The model under review builds one solid part; all positions refer to its coordinate system, in mm. Face numbers are marked on the shaded views. A direction names the side the tool comes from. Round coordinates to 2 decimals unless told otherwise and drop trailing zeros. Order: outer loops, then holes, each group sorted by start corner. A loop starts at its lowest first (then second) coordinate and runs counter-clockwise, first axis right, second up. Notation, with made-up numbers: M -40,87 L 14,87 A32 cw 14,117 Z; hole C -19.5,18 d4. An arc over 180 degrees is marked long. Answer as a JSON object with one key per item and string values. Group by question number.
1. Clearance check with flat-ended pins moving along their axes: P1, Ø1, axis at y = 12, z = 11.5, coming from the -X side; P2, Ø5, axis at x = -23.5, z = 8, coming from the +Y side; P3, Ø1.5, axis at y = -3, z = 7, coming from the +X side. State where each tip first meets the part, or that it passes through.
2. Add section B-B on y = -21. State the section outline as (x, z) points.
3. Add section C-C on x = 22.5. State the section outline as (y, z) points, and give its area (3 significant figures).
4. Add section A-A on z = 4. State the section outline as (x, y) points, and give its area (3 significant figures).
5. Mouldability with a two-part tool opening along X and no side actions: class the marked faces 3, 4 and 5 as released by +X, released by -X, zero draft, split by the parting line, or undercut.
6. Machinability: for the marked faces 1 and 2, which of the approach directions +Z, -Z, +X, -X, +Y, -Y give a long, thin tool a straight path to every point of the face, cutting with its end or side? Answer none if there is none.
7. To check wall thickness, follow probe 1 along X at (y, z) = (-23.7, 16); probe 2 along Z at (x, y) = (22.5, -22); probe 3 along X at (y, z) = (5.5, 8.5). State the ranges of each line that lie inside material, in increasing order. Write a range as [from, to].
8. Add section D-D on x = 0. State the section outline as (y, z) points, and give its area (3 significant figures).
```python
from build123d import *

# Parameters (mm, degrees)
SKETCH_1_W          = 35
SKETCH_1_H          = 50
EXTRUDE_1_DEPTH     = 20
SKETCH_2_W          = 20
SKETCH_2_H          = 5
EXTRUDE_2_DEPTH     = 10
SKETCH_3_W          = 20
SKETCH_3_H          = 5
EXTRUDE_3_DEPTH     = 10
SKETCH_4_R          = 12
CUT_EXTRUDE_1_DEPTH = 20
SKETCH_5_R          = 1.5
CUT_EXTRUDE_2_DEPTH = 5
SKETCH_6_R          = 1.5
CUT_EXTRUDE_3_DEPTH = 5
SKETCH_7_R          = 1.5
CUT_EXTRUDE_4_DEPTH = 5
SKETCH_8_R          = 1.5
CUT_EXTRUDE_5_DEPTH = 5


with BuildPart() as part:
    # Эскиз1 → Бобышка-Вытянуть1 (new body)
    with BuildSketch(Plane.XY):
        Rectangle(SKETCH_1_W, SKETCH_1_H)
    extrude(amount=EXTRUDE_1_DEPTH)

    # Эскиз2 → Бобышка-Вытянуть2 (add)
    with BuildSketch(Plane(origin=(17.5, 0, 0), x_dir=(0, 0, -1), z_dir=(1, 0, 0))):
        with Locations((-10, -22.5)):
            Rectangle(SKETCH_2_W, SKETCH_2_H)
    extrude(amount=EXTRUDE_2_DEPTH)

    # Эскиз3 → Бобышка-Вытянуть3 (add)
    with BuildSketch(Plane.ZY.offset(17.5)):
        with Locations((10, -22.5)):
            Rectangle(SKETCH_3_W, SKETCH_3_H)
    extrude(amount=EXTRUDE_3_DEPTH)

    # Эскиз4 → Вырез-Вытянуть1 (cut)
    with BuildSketch(Plane(origin=(0, 0, 0), x_dir=(-1, 0, 0), z_dir=(0, 0, -1))):
        with Locations((0, 5)):
            Circle(SKETCH_4_R)
    extrude(amount=-CUT_EXTRUDE_1_DEPTH, mode=Mode.SUBTRACT)

    # Эскиз5 → Вырез-Вытянуть2 (cut)
    with BuildSketch(Plane(origin=(0, -20, 0), x_dir=(1, 0, 0), z_dir=(0, 1, 0))):
        with Locations((-22.5, -4)):
            Circle(SKETCH_5_R)
    extrude(amount=-CUT_EXTRUDE_2_DEPTH, mode=Mode.SUBTRACT)

    # Эскиз6 → Вырез-Вытянуть3 (cut)
    with BuildSketch(Plane(origin=(0, -20, 0), x_dir=(1, 0, 0), z_dir=(0, 1, 0))):
        with Locations((-22.5, -16)):
            Circle(SKETCH_6_R)
    extrude(amount=-CUT_EXTRUDE_3_DEPTH, mode=Mode.SUBTRACT)

    # Эскиз7 → Вырез-Вытянуть4 (cut)
    with BuildSketch(Plane(origin=(0, -20, 0), x_dir=(1, 0, 0), z_dir=(0, 1, 0))):
        with Locations((22.5, -4)):
            Circle(SKETCH_7_R)
    extrude(amount=-CUT_EXTRUDE_4_DEPTH, mode=Mode.SUBTRACT)

    # Эскиз8 → Вырез-Вытянуть5 (cut)
    with BuildSketch(Plane(origin=(0, -20, 0), x_dir=(1, 0, 0), z_dir=(0, 1, 0))):
        with Locations((22.5, -16)):
            Circle(SKETCH_8_R)
    extrude(amount=-CUT_EXTRUDE_5_DEPTH, mode=Mode.SUBTRACT)


solid = part.part
```
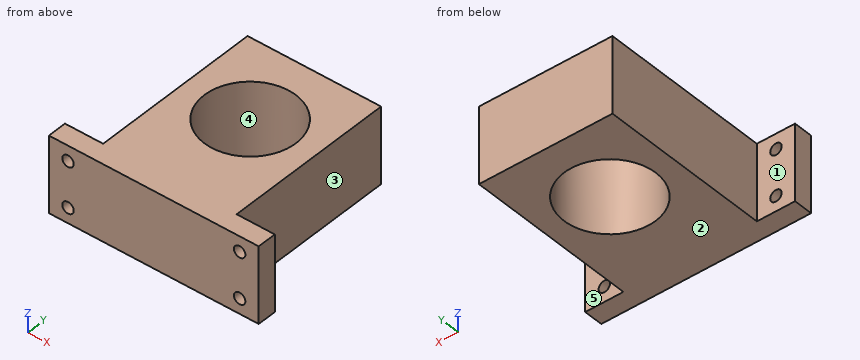
Recorded:
{
 "1": {"P1": "stops at x = -17.5", "P2": "stops at y = -20", "P3": "stops at x = 17.5"},
 "2": {"outline": "M -27.5,0 L 27.5,0 L 27.5,20 L -27.5,20 Z; hole C -22.5,4 d3; hole C -22.5,16 d3; hole C 22.5,4 d3; hole C 22.5,16 d3"},
 "3": {"outline": "M -25,0 L -20,0 L -20,2.5 L -25,2.5 Z; M -25,5.5 L -20,5.5 L -20,14.5 L -25,14.5 Z; M -25,17.5 L -20,17.5 L -20,20 L -25,20 Z", "area": "70.0 mm²"},
 "4": {"outline": "M -27.5,-25 L -24,-25 L -24,-20 L -27.5,-20 Z; M -21,-25 L 21,-25 L 21,-20 L 17.5,-20 L 17.5,25 L -17.5,25 L -17.5,-20 L -21,-20 Z; M 24,-25 L 27.5,-25 L 27.5,-20 L 24,-20 Z; hole C 0,5 d24", "area": "1,370 mm²"},
 "5": {"face 3": "released by +X", "face 4": "undercut", "face 5": "zero draft"},
 "6": {"face 1": "+Z, -Z, -X, +Y", "face 2": "-Z, +X, -X, +Y, -Y"},
 "7": {"probe 1": "x = [-27.5, -24], [-21, 21], [24, 27.5]", "probe 2": "z = [0, 2.5], [5.5, 14.5], [17.5, 20]", "probe 3": "x = [-17.5, -11.99], [11.99, 17.5]"},
 "8": {"outline": "M -25,0 L -7,0 L -7,20 L -25,20 Z; M 17,0 L 25,0 L 25,20 L 17,20 Z", "area": "520 mm²"}
}
